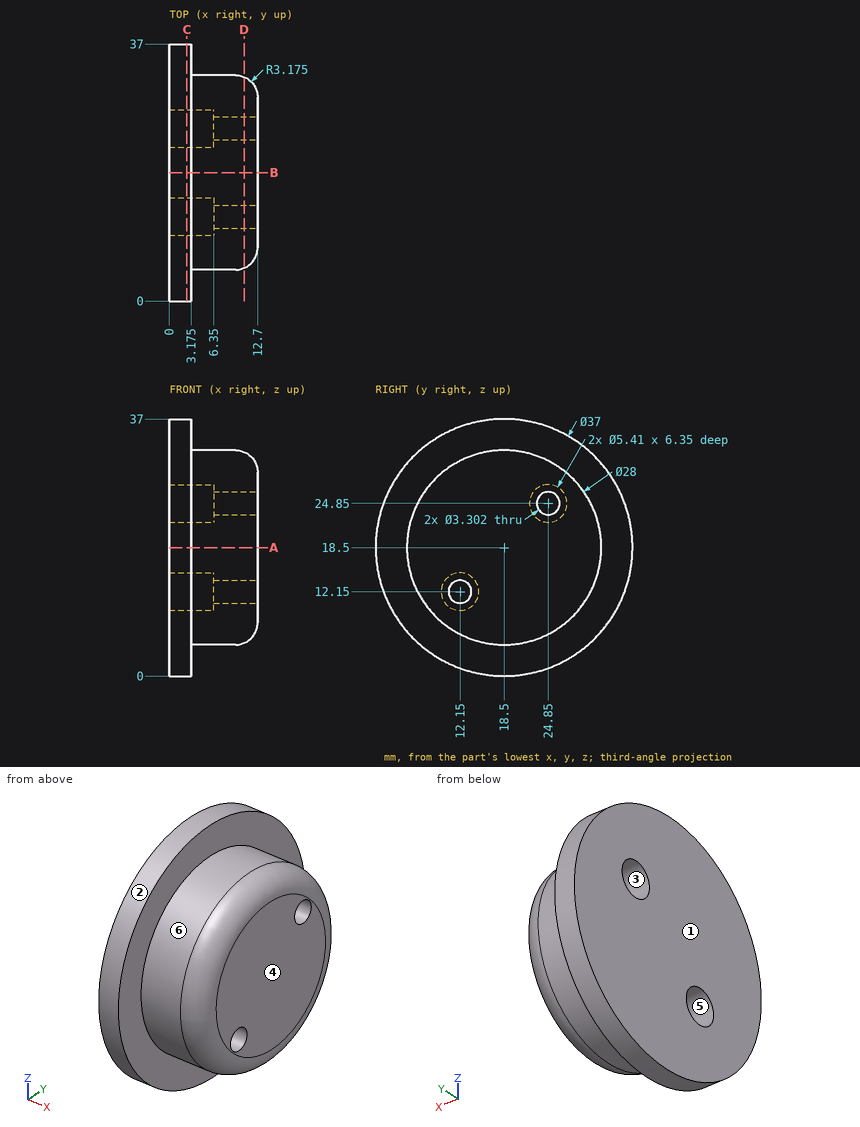
Source: three-view drawing plus pictorial views. Frame: mm from the lowest corner of the part. A direction names the side the tool comes from. Coordinates: 2 decimals unless noted, no trailing zeros. Order: outer loops, then holes, each group sorted by start corner. A loop starts at its lowest first (then second) coordinate and runs counter-clockwise, first axis right, second up. Notation, with made-up numbers: (51.25, 83.5) -> (85.25, 83.5) arc R31 cw to (85.25, 107.5) -> close; hole circle Ø2 at (67, 86). An arc over 180 degrees is marked (long way). Write item = value, one per line.
(1) Cut plane C-C on x = 2.5. Count the separate pieces of the cut face and the enclosed holes in it, plus the area to 3 significant figures.
Solved:
separate_pieces = 1
enclosed_holes = 2
area = 1,030 mm²
(2) Cut plane D-D on x = 10.75. Return loops of the section in (y, z).
Solved:
outline = circle Ø27.51 at (18.5, 18.5); hole circle Ø3.3 at (12.15, 12.15); hole circle Ø3.3 at (24.85, 24.85)
(3) Cut plane A-A on z = 18.5. Return loops of the section in (x, y) (3 decimals), plus the area to 3 significant figures.
Solved:
outline = (0, 0) -> (3.175, 0) -> (3.175, 4.5) -> (9.525, 4.5) arc R3.175 ccw to (12.7, 7.675) -> (12.7, 29.325) arc R3.175 ccw to (9.525, 32.5) -> (3.175, 32.5) -> (3.175, 37) -> (0, 37) -> close
area = 380 mm²
(4) Line query: line 1 (Y direction, x = 4.75, z = 24.85) (1 decimal); line 2 (X direction, y = 35, z = 10.5) (3 decimals); line 3 (Y direction, x = 0.75, z = 25). Output: solid intervals per line, ascending.
Solved:
line_1 = 6 to 22.1, 27.6 to 31
line_2 = 0 to 3.175
line_3 = 1.18 to 22.15, 27.55 to 35.82
(5) Pin query (flat end, axial travel): pin 1 Ø5 at (x, z) = (11, 13) entering from -Y; pin 2 Ø6 at (x, y) = (7.5, 27) entering from -Z; pin 3 Ø5 at (x, y) = (6.5, 17) entering from -Z. Return the tip coordinate at first contact, or that it passes through.
Solved:
pin_1 = 4.91
pin_2 = 5.63
pin_3 = 4.5
(6) Pull-direction query (Z, two-part tool) for the marked faces 1, 2 and 3; classes: pulls with the +Z half, pulls with the -Z half, needs draft (parallel to the pull), parting line crosses it, or undercut.
Solved:
face_1 = needs draft
face_2 = parting line crosses it
face_3 = undercut
(7) Access query for the marked faces 4, 5 and 6. Directions: +Z, -Z, +X, -X, +Y, -Y. A direction counts if a zero-diameter tool reaches every point of the face in a straight line with its end or side. Return the directions, or none.
Solved:
face_4 = +Z, -Z, +X, +Y, -Y
face_5 = -X
face_6 = +X
